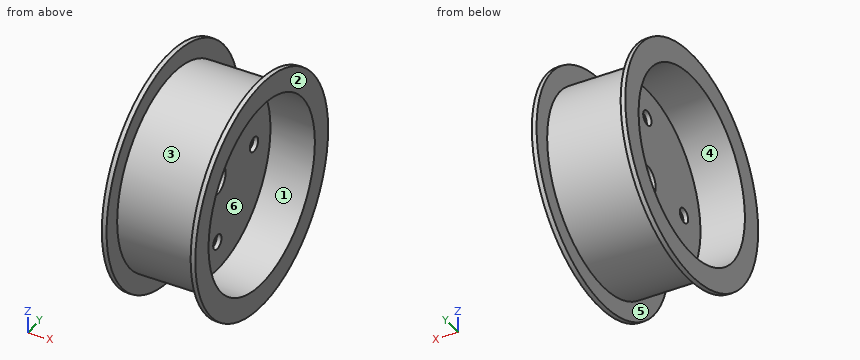
from build123d import *

# Parameters (mm, degrees)
CUT_EXTRUDE1_REACH = 28.67
SKETCH2_R          = 3.96875
SKETCH2_R_2        = 7.9375


with BuildPart() as part:
    # Sketch1 → Revolve1 (revolve)
    with BuildSketch(Plane.XY):
        Polygon((0, 0), (-1.27, 0), (-1.27, 50.8), (-25.4, 50.8), (-25.4, 63.5), (-22.86, 63.5), (-22.86, 53.34), (0, 53.34), (0, 50.8), align=None)
    revolve1 = revolve(axis=Axis((0, 0, 0), (-1, 0, 0)))

    # Mirror1: Revolve1 across plane
    add(revolve1.mirror(Plane(origin=(0, 0, 0), x_dir=(0, 0, 1), z_dir=(1, 0, 0))))

    # Sketch2 → Cut-Extrude1 (cut, up to next)
    with BuildSketch(Plane(origin=(1.27, 0, 0), x_dir=(0, 0, -1), z_dir=(1, 0, 0)), mode=Mode.PRIVATE) as cut_extrude1_sk1:
        with Locations((35.052, 0)):
            Circle(SKETCH2_R)
    cut_extrude1_tool1 = extrude(cut_extrude1_sk1.sketch, amount=-CUT_EXTRUDE1_REACH, mode=Mode.PRIVATE) & part.part
    add(cut_extrude1_tool1.solids().sort_by_distance((1.27, 0, -35.052))[0], mode=Mode.SUBTRACT)
    # Sketch2 → Cut-Extrude1 (cut, up to next)
    with BuildSketch(Plane(origin=(1.27, 0, 0), x_dir=(0, 0, -1), z_dir=(1, 0, 0)), mode=Mode.PRIVATE) as cut_extrude1_sk2:
        with Locations((0, 35.052)):
            Circle(SKETCH2_R)
    cut_extrude1_tool2 = extrude(cut_extrude1_sk2.sketch, amount=-CUT_EXTRUDE1_REACH, mode=Mode.PRIVATE) & part.part
    add(cut_extrude1_tool2.solids().sort_by_distance((1.27, 35.052, 0))[0], mode=Mode.SUBTRACT)
    # Sketch2 → Cut-Extrude1 (cut, up to next)
    with BuildSketch(Plane(origin=(1.27, 0, 0), x_dir=(0, 0, -1), z_dir=(1, 0, 0)), mode=Mode.PRIVATE) as cut_extrude1_sk3:
        with Locations((0, -35.052)):
            Circle(SKETCH2_R)
    cut_extrude1_tool3 = extrude(cut_extrude1_sk3.sketch, amount=-CUT_EXTRUDE1_REACH, mode=Mode.PRIVATE) & part.part
    add(cut_extrude1_tool3.solids().sort_by_distance((1.27, -35.052, 0))[0], mode=Mode.SUBTRACT)
    # Sketch2 → Cut-Extrude1 (cut, up to next)
    with BuildSketch(Plane(origin=(1.27, 0, 0), x_dir=(0, 0, -1), z_dir=(1, 0, 0)), mode=Mode.PRIVATE) as cut_extrude1_sk4:
        with Locations((-35.052, 0)):
            Circle(SKETCH2_R)
    cut_extrude1_tool4 = extrude(cut_extrude1_sk4.sketch, amount=-CUT_EXTRUDE1_REACH, mode=Mode.PRIVATE) & part.part
    add(cut_extrude1_tool4.solids().sort_by_distance((1.27, 0, 35.052))[0], mode=Mode.SUBTRACT)
    # Sketch2 → Cut-Extrude1 (cut, up to next)
    with BuildSketch(Plane(origin=(1.27, 0, 0), x_dir=(0, 0, -1), z_dir=(1, 0, 0)), mode=Mode.PRIVATE) as cut_extrude1_sk5:
        Circle(SKETCH2_R_2)
    cut_extrude1_tool5 = extrude(cut_extrude1_sk5.sketch, amount=-CUT_EXTRUDE1_REACH, mode=Mode.PRIVATE) & part.part
    add(cut_extrude1_tool5.solids().sort_by_distance((1.27, 0, 0))[0], mode=Mode.SUBTRACT)


solid = part.part
Input: part model. Units: mm. Frame: model coordinates. Face numbers are marked on the shaded views. A direction names the side the tool comes from. Round coordinates to 2 decimals unless told otherwise and drop trailing zeros. Loops run counter-clockwise (first coordinate to the right, second up) from the corner with the lowest first, then second, coordinate; pieces in that order, holes last. Notation, with made-up numbers: (-16, 16) -> (16, 16) arc R35 ccw to (16, 54) -> close; hole circle Ø9 at (71.25, 74.5). An arc over 180 degrees is marked (long way). Answer as a JSON object with one key per item and string values. Group by question number.
1) Pin query (flat end, axial travel): pin 1 (3 mm diameter, centred on y = 12, z = -6.5, fed in from -X); pin 2 (12 mm diameter, centred on x = -17.5, y = 11, fed in from -Z); pin 3 (8 mm diameter, centred on x = -10, y = -10, fed in from -Z). Return the tip coordinate at first contact, or that it passes through.
2) Ray query, L1, parallel to Y at x = 0.5, z = 0; L2, parallel to Y at x = -12, z = 0; L3, parallel to X at y = -45, z = -42.5. Return the intervals inside material, ascending.
3) Draft query along Z for the marked faces 1, 2 and 3. Return one class per face: +Z half, -Z half, draft (parallel to the pull), parting line (faces both ways), or undercut.
4) Section query A-A on y = 0. State how many separate pieces and enclosed holes the cut face has, plus the area to 3 significant figures.
5) Section query C-C on x = 19. Output: boundary loops of the cut face in (y, z).
6) Section query D-D on y = 26. Output: boundary loops of the cut face in (x, z).
7) Reachability of the marked faces 4, 5 and 6 from +Z, -Z, +X, -X, +Y, -Y: full face, straight path, thin tool, end or side. Return the list, or none.
Reply:
{
 "1": {"pin 1": "stops at x = -1.27", "pin 2": "stops at z = -62.95", "pin 3": "stops at z = -53"},
 "2": {"L1": "y = -53.34 to -39.02, -31.08 to -7.94, 7.94 to 31.08, 39.02 to 53.34", "L2": "y = -53.34 to -50.8, 50.8 to 53.34", "L3": "x = -25.4 to -22.86, 22.86 to 25.4"},
 "3": {"face 1": "undercut", "face 2": "draft", "face 3": "parting line"},
 "4": {"separate pieces": "4", "enclosed holes": "0", "area": "539 mm2"},
 "5": {"outline": "circle Ø106.68 at (0, 0); hole circle Ø101.6 at (0, 0)"},
 "6": {"outline": "(-25.4, -57.93) -> (-22.86, -57.93) -> (-22.86, -46.57) -> (22.86, -46.57) -> (22.86, -57.93) -> (25.4, -57.93) -> (25.4, -43.64) -> (1.27, -43.64) -> (1.27, 43.64) -> (25.4, 43.64) -> (25.4, 57.93) -> (22.86, 57.93) -> (22.86, 46.57) -> (-22.86, 46.57) -> (-22.86, 57.93) -> (-25.4, 57.93) -> (-25.4, 43.64) -> (-1.27, 43.64) -> (-1.27, -43.64) -> (-25.4, -43.64) -> close"},
 "7": {"face 4": "-X", "face 5": "none", "face 6": "+X"}
}
